Geometry: final body of the model. Coordinates: model frame, mm. Give positions to 0.01 mm unless a question says otherwise; leave off trailing zeros. Loops run counter-clockwise (first coordinate to the right, second up) from the corner with the lowest first, then second, coordinate; pieces in that order, holes last.
from build123d import *

# Parameters (mm, degrees)
BOSS_EXTRUDE2_DEPTH = 15.24


with BuildPart() as part:
    # Sketch1 → Boss-Extrude2 (new body)
    with BuildSketch(Plane(origin=(0, 0, 0), x_dir=(1, 0, 0), z_dir=(0, 1, 0))):
        with BuildLine():
            Line((-6.35, 115.371368334), (6.35, 115.371368334))
            Line((6.35, 115.371368334), (6.35, 101.401368334))
            ThreePointArc((6.35, 101.401368334), (71.842048969, 71.842048969), (101.401368334, 6.35))
            Line((101.401368334, 6.35), (115.371368334, 6.35))
            Line((115.371368334, 6.35), (115.371368334, -3.175))
            Line((115.371368334, -3.175), (115.371368334, -6.35))
            Line((115.371368334, -6.35), (101.401368334, -6.35))
            ThreePointArc((101.401368334, -6.35), (71.842048969, -71.842048969), (6.35, -101.401368334))
            Line((6.35, -101.401368334), (6.35, -115.371368334))
            Line((6.35, -115.371368334), (-6.35, -115.371368334))
            Line((-6.35, -115.371368334), (-6.35, -101.401368334))
            ThreePointArc((-6.35, -101.401368334), (-71.842048969, -71.842048969), (-101.401368334, -6.35))
            Line((-101.401368334, -6.35), (-115.371368334, -6.35))
            Line((-115.371368334, -6.35), (-115.371368334, 6.35))
            Line((-115.371368334, 6.35), (-101.401368334, 6.35))
            ThreePointArc((-101.401368334, 6.35), (-71.842048969, 71.842048969), (-6.35, 101.401368334))
            Line((-6.35, 101.401368334), (-6.35, 115.371368334))
        make_face()
    extrude(amount=BOSS_EXTRUDE2_DEPTH)


solid = part.part
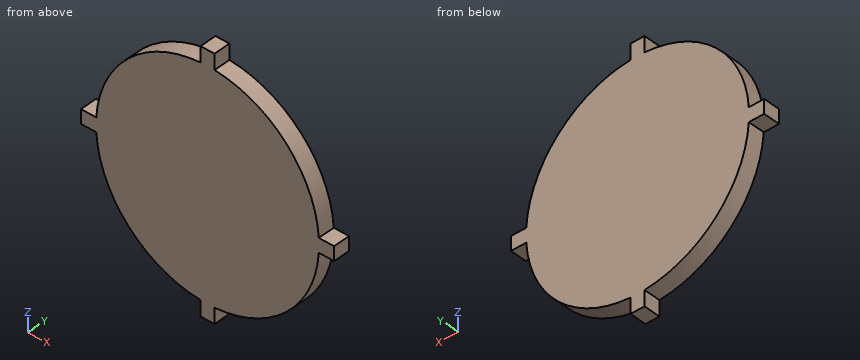
Item 1: Section query A-A on y = 3.5. Return loops of the section in (x, z), plus the area to 3 significant figures.
Values follow:
outline: (-115.37, -6.35) - (-101.4, -6.35) arc R101.6 ccw to (-6.35, -101.4) - (-6.35, -115.37) - (6.35, -115.37) - (6.35, -101.4) arc R101.6 ccw to (101.4, -6.35) - (115.37, -6.35) - (115.37, 6.35) - (101.4, 6.35) arc R101.6 ccw to (6.35, 101.4) - (6.35, 115.37) - (-6.35, 115.37) - (-6.35, 101.4) arc R101.6 ccw to (-101.4, 6.35) - (-115.37, 6.35) - close
area: 33,100 mm2
Item 2: Pin query (flat end, axial travel): pin 1 (4 mm diameter, centred on y = 11, z = -64.5, fed in from -X); pin 2 (3 mm diameter, centred on y = 7, z = -58.5, fed in from -X); pin 3 (2 mm diameter, centred on y = 5, z = -22.5, fed in from -X). Return the tip coordinate at first contact, or that it passes through.
Values follow:
pin 1: stops at x = -80.1
pin 2: stops at x = -84.1
pin 3: stops at x = -99.3
Item 3: Section query B-B on x = 34.5. Return loops of the section in (y, z), plus the area to 3 significant figures.
Values follow:
outline: (0, -95.56) - (15.24, -95.56) - (15.24, 95.56) - (0, 95.56) - close
area: 2,910 mm2
Item 4: Section query C-C on z = 59.5. Return loops of the section in (x, y).
Values follow:
outline: (-82.35, 0) - (82.35, 0) - (82.35, 15.24) - (-82.35, 15.24) - close
Item 5: Ray query, probe 1 along Z at (x, y) = (-104.5, 2.25); probe 2 along X at (y, z) = (3.5, -20); probe 3 along Z at (x, y) = (92.5, 13). Return the intervals inside material, ascending.
Values follow:
probe 1: z = -6.35 to 6.35
probe 2: x = -99.61 to 99.61
probe 3: z = -42.03 to 42.03
